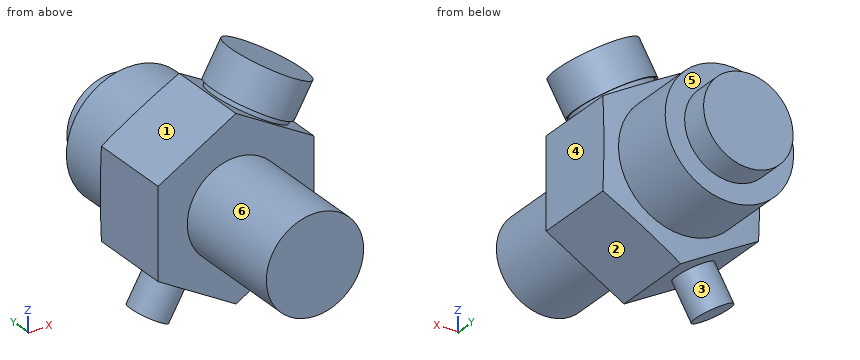
from build123d import *

# Parameters (mm, degrees)
SKETCH2_R                = 31.284897101
CUT_EXTRUDE2_DEPTH       = 58.150000089
SKETCH3_R                = 3.175
BOSS_EXTRUDE1_DEPTH      = 6.35
SKETCH4_R                = 6.35
BOSS_EXTRUDE3_DEPTH      = 6.35
BOSS_EXTRUDE4_DEPTH      = 0.508
BOSS_EXTRUDE4_DEPTH_BACK = 5.588
SKETCH5_R                = 6.858
SKETCH5_R_2              = 6.604
SKETCH5_3_R              = 6.604
BOSS_EXTRUDE5_DEPTH      = 0.508
SKETCH6_R                = 7.3025
BOSS_EXTRUDE6_DEPTH      = 4.572


with BuildPart() as part:
    # Sketch1 → Revolve1 (revolve)
    with BuildSketch(Plane(origin=(0, 0, 0), x_dir=(0, 0, -1), z_dir=(1, 0, 0))):
        with BuildLine():
            Line((10.4775, 33.195692203), (10.4775, 44.45))
            Line((10.4775, 44.45), (0, 44.45))
            Line((0, 44.45), (0, 0))
            Line((0, 0), (7.9375, 0))
            Line((7.9375, 0), (7.9375, 19.05))
            Line((7.9375, 19.05), (25.4, 19.05))
            Line((25.4, 19.05), (25.4, 30.511567858))
            ThreePointArc((25.4, 30.511567858), (17.996597132, 32.175233549), (10.4775, 33.195692203))
        make_face()
    revolve(axis=Axis((0, 0, 0), (0, 1, 0)))

    # Sketch2 → Cut-Extrude2 (cut, through all)
    with BuildSketch(Plane(origin=(0, 0, 0), x_dir=(1, 0, 0), z_dir=(0, 1, 0))):
        Circle(SKETCH2_R)
        Polygon((-12.7, 7.332348419), (0, 14.664696837), (12.7, 7.332348419), (12.7, -7.332348419), (0, -14.664696837), (-12.7, -7.332348419), align=None, mode=Mode.SUBTRACT)
    extrude(amount=CUT_EXTRUDE2_DEPTH, mode=Mode.SUBTRACT)

    # Sketch3 → Boss-Extrude1 (add)
    with BuildSketch(Plane(origin=(-6.35, 0, -10.998522628), x_dir=(-0.8660254037844386, 0, 0.5000000000000002), z_dir=(-0.5000000000000001, 0, -0.8660254037844385))):
        with Locations(Location((0, 26.307433584, 0), (0, 0, 180))):
            Circle(SKETCH3_R)
    extrude(amount=BOSS_EXTRUDE1_DEPTH)

    # Sketch4 → Boss-Extrude3 (add)
    with BuildSketch(Plane(origin=(6.35, 0, 10.998522628), x_dir=(0.8660254037844406, 0, -0.49999999999999684), z_dir=(0.49999999999999684, 0, 0.8660254037844406))):
        with Locations(Location((0, 26.044781418, 0), (0, 0, 180))):
            Circle(SKETCH4_R)
    extrude(amount=BOSS_EXTRUDE3_DEPTH)



with BuildPart() as body_2:
    # Sketch5 → Boss-Extrude4 (new, two sides: drawn at the far end of the back side and taken through both)
    with BuildSketch(Plane(origin=(9.525, 0, 16.497783942), x_dir=(0.8660254037844405, 0, -0.49999999999999695), z_dir=(0.4999999999999969, 0, 0.8660254037844404)).offset(-BOSS_EXTRUDE4_DEPTH_BACK)):
        with Locations((0, 26.044781418)):
            Circle(SKETCH5_R)
        with Locations((0, 26.044781418)):
            Circle(SKETCH5_R_2, mode=Mode.SUBTRACT)
    extrude(amount=BOSS_EXTRUDE4_DEPTH + BOSS_EXTRUDE4_DEPTH_BACK)


with BuildPart() as part_1:
    add(part.part)

    add(body_2.part)  # Boss-Extrude5 merges body 2
    # Sketch5_3 → Boss-Extrude5 (add)
    with BuildSketch(Plane(origin=(9.525, 0, 16.497783942), x_dir=(0.8660254037844405, 0, -0.49999999999999695), z_dir=(0.4999999999999969, 0, 0.8660254037844404))):
        with Locations((0, 26.044781418)):
            Circle(SKETCH5_3_R)
    extrude(amount=BOSS_EXTRUDE5_DEPTH)

    # Sketch6 → Boss-Extrude6 (add)
    with BuildSketch(Plane(origin=(0, 44.45, 0), x_dir=(1, 0, 0), z_dir=(0, 1, 0))):
        with Locations(Location((0, 0, 0), (0, 0, 270))):
            Circle(SKETCH6_R)
    extrude(amount=BOSS_EXTRUDE6_DEPTH)


solid = part_1.part
Model file for the job. Use its own axes, mm. Face numbers are marked on the shaded views. A direction names the side the tool comes from. Give positions to 0.01 mm unless a question says otherwise; leave off trailing zeros. Loops run counter-clockwise (first coordinate to the right, second up) from the corner with the lowest first, then second, coordinate; pieces in that order, holes last. Notation, with made-up numbers: (-11.5, 11) -> (22.5, 11) arc R28 ccw to (22.5, 44) -> close; hole circle Ø10 at (82, 51). An arc over 180 degrees is marked (long way). Use a Markdown table: item, result. Add a question column.
(1) Mould opens along X. For the marked faces 1, 2 and 3 say: +X half, -X half, draft (parallel to the pull), parting line (faces both ways), or undercut.
(2) Slice it at A-A on y = 10.5. List the corners of the cut face in (x, z) (1 decimal), and give its area (3 significant figures).
(3) Wall check: line 1 along Y through (x, z) = (7.75, 12.5); line 2 along Y through (x, z) = (11.5, 14); line 3 along X through (y, z) = (27.5, -4.5). Give the ranges that are in metal, low to high.
(4) Drop flat-ended pins along their axis: pin 1 Ø8 at (x, z) = (-2, -14) entering from +Y; pin 2 Ø2 at (x, z) = (9.5, 10.5) entering from +Y; pin 3 Ø4 at (x, y) = (10.5, 42) entering from +Z; pin 4 Ø4 at (x, z) = (-8, 14) entering from +Y. Give the stop position or say it passes through.
(5) Tool access for the marked faces 4, 5 and 6: list every direction of +Z, -Z, +X, -X, +Y, -Y with a clear straight run to the whole face (end or side of a thin tool).
Filled sheet:
| question | item | result |
|---|---|---|
| 1 | face 1 | -X half |
| 1 | face 2 | +X half |
| 1 | face 3 | undercut |
| 2 | outline | circle Ø15.9 at (0, 0) |
| 2 | area | 198 mm2 |
| 3 | line 1 | 19.2 to 19.46, 19.71 to 32.38, 32.63 to 32.89 |
| 3 | line 2 | 19.86 to 20.14, 20.43 to 31.66, 31.95 to 32.23 |
| 3 | line 3 | -12.7 to 12.7 |
| 4 | pin 1 | y = 44.45 |
| 4 | pin 2 | y = 32.61 |
| 4 | pin 3 | z = 6.13 |
| 4 | pin 4 | through |
| 5 | face 4 | -Z, +X, +Y, -Y |
| 5 | face 5 | +Y |
| 5 | face 6 | -Y |
